Design review of the part shown in the three views and the two pictorial views. Dimensions are in mm from the part's minimum x, y and z. A direction names the side the tool comes from. Round coordinates to 2 decimals unless told otherwise and drop trailing zeros. Loops run counter-clockwise (first coordinate to the right, second up) from the corner with the lowest first, then second, coordinate; pieces in that order, holes last. Notation, with made-up numbers: M 26,10.5 L 82,10.5 A22 ccw 82,32.5 Z; hole C 11,26 d4. An arc over 180 degrees is marked long. One line per question, with ' | ' between items. Start each with the question number.
1) We need section B-B (y = 32). Give the boundary of the cut face in (x, z) (1 decimal).
2) For pin 1 Ø6 at (x, y) = (146, 31) entering from -Z (1 decimal); pin 2 Ø3 at (y, z) = (64.5, 68.5) entering from +X; pin 3 Ø10 at (x, y) = (63, 54) entering from +Z; pin 4 Ø3 at (y, z) = (26.5, 56) entering from -X, all flat-tipped, find the tip position at first contact; note any pin that passes through.
3) We need section A-A (z = 45). Give the boundary of the cut face in (x, y).
4) For the marked faces 1 and 2, list the 3-axis set-ups (+Z, -Z, +X, -X, +Y, -Y) from which the entire face can be reached by the end or side of a thin tool; tool diameter is ignored.
5) We need section C-C (x = 32). Give the boundary of the cut face in (y, z), and give its area (3 significant figures).
6) For probe 1 along Y at (x, z) = (120, 45); probe 2 along Z at (x, y) = (254.5, 38); probe 3 along Y at (x, z) = (250, 35), list the stretches that pass through material, from the lowest coordinate up. Write a range as from..to.
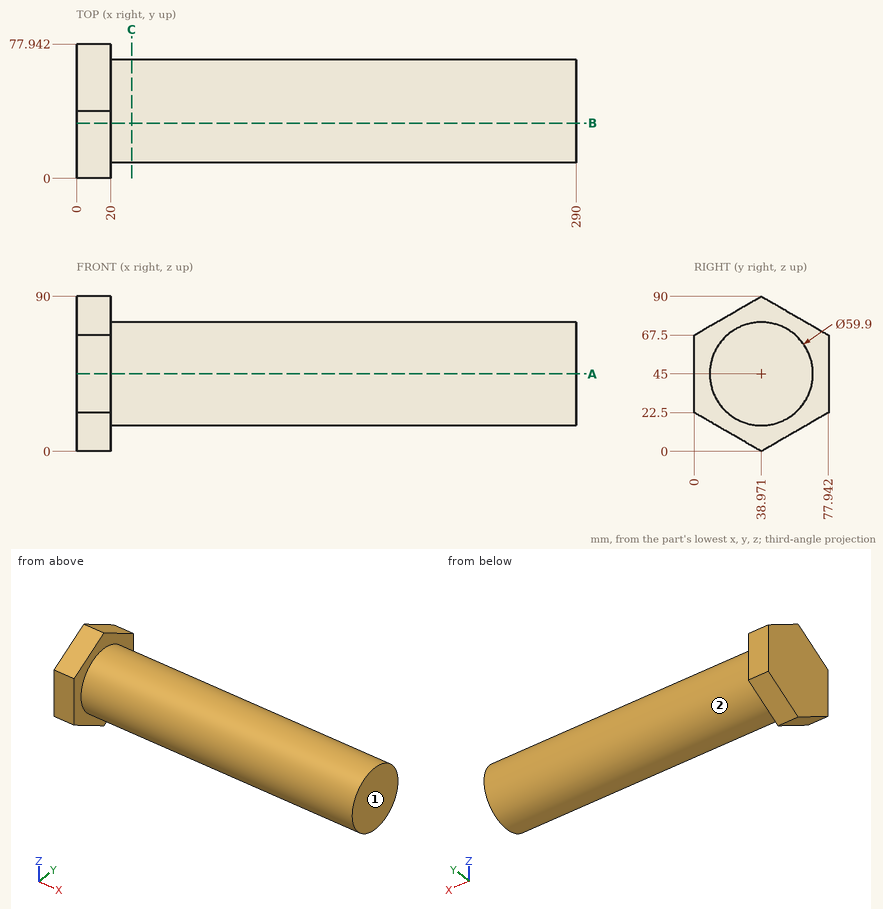
Answers below:
1) outline: M 0,4 L 20,4 L 20,15.9 L 290,15.9 L 290,74.1 L 20,74.1 L 20,86 L 0,86 Z
2) pin 1: z = 15.5 | pin 2: x = 20 | pin 3: z = 73.22 | pin 4: x = 0
3) outline: M 0,0 L 20,0 L 20,9.02 L 290,9.02 L 290,68.92 L 20,68.92 L 20,77.94 L 0,77.94 Z
4) face 1: +Z, -Z, +X, +Y, -Y | face 2: +X
5) outline: C 38.97,45 d59.9 | area: 2,820 mm^2
6) probe 1: 9.02..68.92 | probe 2: 15.07..74.93 | probe 3: 10.74..67.2
